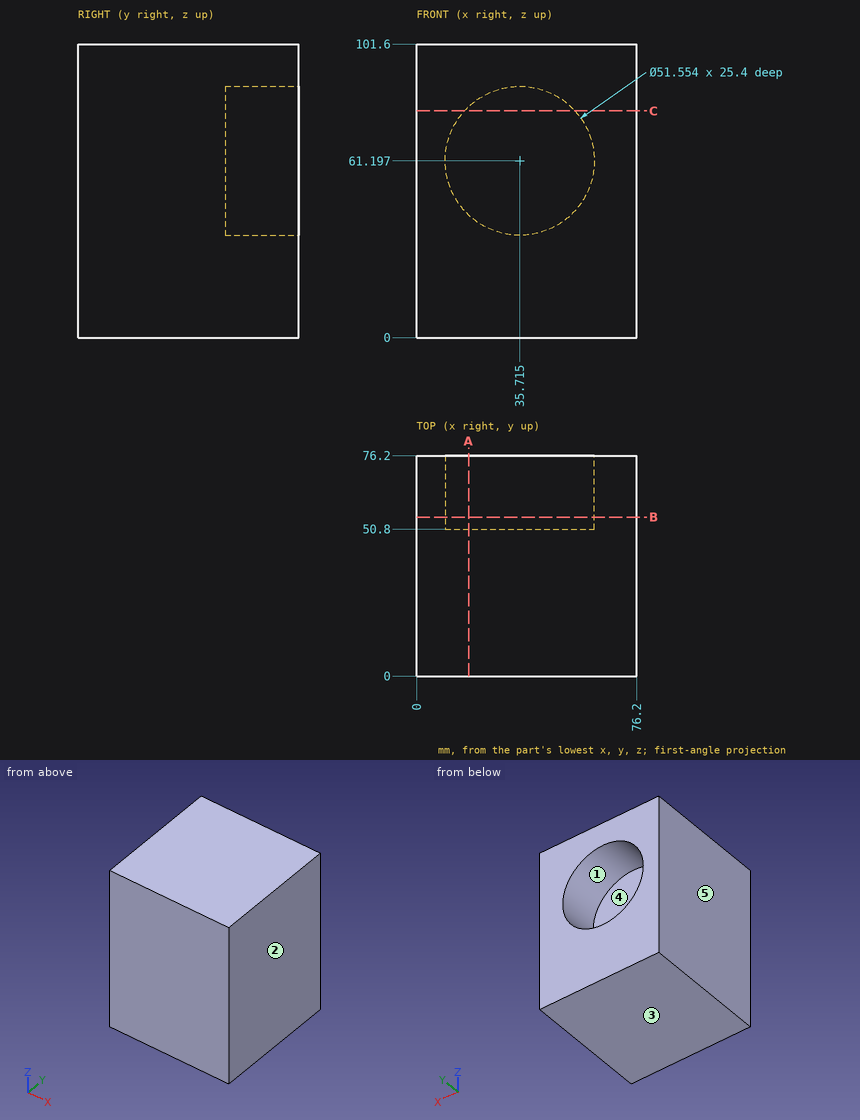
Verification items for this drawing (mm, ordinates from the low corner). A direction names the side the tool comes from. Give positions to 0.01 mm unless a question says otherwise; leave off trailing zeros. Loops run counter-clockwise (first coordinate to the right, second up) from the corner with the lowest first, then second, coordinate; pieces in that order, holes last.
(1) Section check C-C on z = 78.5. Record the cut outline in (x, y), then the cut area to 3 significant figures.
From the geometry:
outline: (0, 0) - (76.2, 0) - (76.2, 76.2) - (54.82, 76.2) - (54.82, 50.8) - (16.61, 50.8) - (16.61, 76.2) - (0, 76.2) - close
area: 4,840 mm2
(2) Thickness scan on L1, parallel to Z at x = 43, y = 66.5; L2, parallel to Z at x = 15, y = 59.5 (1 decimal); L3, parallel to Y at x = 43, z = 71. Record the ranges inside material, lowest first.
From the geometry:
L1: z = 0 to 36.47, 85.92 to 101.6
L2: z = 0 to 45.9, 76.5 to 101.6
L3: y = 0 to 50.8
(3) Release check for a two-part mould opening along X. For the marked faces 1, 2 and 3 record: released by +X, released by -X, zero draft, split by the parting line, or undercut.
From the geometry:
face 1: undercut
face 2: released by +X
face 3: zero draft
(4) Set-up check for the marked faces 4 and 5: record each of +Z, -Z, +X, -X, +Y, -Y from which the full face is reachable in a straight line by a thin tool's end or side.
From the geometry:
face 4: +Y
face 5: +Z, -Z, -X, +Y, -Y
(5) Depth check by flat-ended pin: pin 1 Ø2 at (x, z) = (41.5, 75.5) entering from +Y. Enter the tip coordinate at first touch or a pass-through.
From the geometry:
pin 1: stops at y = 50.8
(6) Section check A-A on x = 18. Record the cut outline in (y, z), then the cut area to 3 significant figures.
From the geometry:
outline: (0, 0) - (76.2, 0) - (76.2, 42.47) - (50.8, 42.47) - (50.8, 79.92) - (76.2, 79.92) - (76.2, 101.6) - (0, 101.6) - close
area: 6,790 mm2
(7) Section check B-B on y = 55. Record the cut outline in (x, z) (1 decimal), then the cut area to 3 significant figures.
From the geometry:
outline: (0, 0) - (76.2, 0) - (76.2, 101.6) - (0, 101.6) - close; hole circle Ø51.6 at (35.7, 61.2)
area: 5,650 mm2
